Design review of the part built by this model. Coordinates are the model's own, in mm. Face numbers are marked on the shaded views. A direction names the side the tool comes from. Give positions to 0.01 mm unless a question says otherwise; leave off trailing zeros. Write each loop counter-clockwise with the first axis right and the second up, starting at its lowest first coordinate (ties: lowest second). Pieces come first, ordered by that corner, then holes. Notation, with made-up numbers: (34.25, 80.5) -> (41.25, 80.5) arc R21 ccw to (41.25, 107.5) -> close; hole circle Ø8 at (-38.75, 61). An arc over 180 degrees is marked (long way). Return JSON: item names as keys, results as strings. Group by question number.
Autodesk Inventor part; units mm, degrees
ref_plane "Work Plane2" through (0, 3.81, 0) normal (0, 1, 0) x (1, 0, 0)
ref_plane "Work Plane1" through (0, -3.81, 0) normal (0, -1, 0) x (1, 0, 0)
ref_plane "Work Plane4" through (1.27, 3.81, -29.21) normal (0, 0, -1) x (-1, 0, 0)
ref_plane "Work Plane2" through (0, 3.81, 0) normal (0, 1, 0) x (1, 0, 0)
sketch "Sketch2" plane through (0, 3.81, 0) normal (0, 1, 0) x (1, 0, 0)
  line L0 (-29.21, 29.21) -> (1.27, 29.21)
  line L1 (1.27, -1.27) -> (-29.21, -1.27)
  line L2 (-29.21, -1.27) -> (-29.21, 29.21)
  line L3 (1.27, -1.27) -> (1.27, 29.21)
  line L4 (-4.8761, 25.94) -> (-25.94, 25.94)
  line L5 (-25.94, 25.94) -> (-25.94, 0)
  line L6 (-25.94, 0) -> (0, 0)
  line L7 (0, 0) -> (0, 21.0639)
  dimension "d3" = 30.48
extrude "Extrusion2" add sketch "Sketch2" along normal blind 11.43
ref_plane "Work Plane1" through (0, -3.81, 0) normal (0, -1, 0) x (1, 0, 0)
ref_plane "Work Plane4" through (1.27, 3.81, -29.21) normal (0, 0, -1) x (-1, 0, 0)
sketch "Sketch6" plane through (1.27, 3.81, -29.21) normal (0, 0, -1) x (-1, 0, 0)
  line L0 (0, 11.43) -> (30.48, 11.43)
  line L1 (0, 11.43) -> (-7.239, 11.43)
  line L2 (-7.239, 11.43) -> (-7.239, 9.9183)
  line L3 (-7.239, 9.9183) -> (0, 9.9183)
  line L4 (0, 9.9183) -> (0, 11.43)
  line L5 (15.24, 11.43) -> (15.24, -7.62) construction
  line L6 (1.27, -7.62) -> (27.21, -7.62) construction
  line L7 (30.48, 11.43) -> (37.719, 11.43)
  line L8 (37.719, 11.43) -> (37.719, 9.9183)
  line L9 (37.719, 9.9183) -> (30.48, 9.9183)
  line L10 (30.48, 9.9183) -> (30.48, 11.43)
  point P0 (1.27, -3.81)
  dimension "d22" = 7.239
extrude "Extrusion6" add sketch "Sketch6" against normal up to surface (30.48 mm away)
ref_plane "Work Plane3" through (0, 15.24, 0) normal (0, 1, 0) x (1, 0, 0)
sketch "Sketch9" plane through (0, 15.24, 0) normal (0, 1, 0) x (1, 0, 0)
  line L0 (8.509, 29.21) -> (8.509, -1.27) construction
  line L1 (8.509, 13.97) -> (-36.449, 13.97) construction
  line L2 (-36.449, 29.21) -> (-36.449, -1.27) construction
  line L3 (-36.449, -1.27) -> (8.509, -1.27) construction
  line L4 (-13.97, -1.27) -> (-13.97, 29.21) construction
  line L5 (-36.449, 29.21) -> (8.509, 29.21) construction
  circle A0 centre (-21.336, 13.97) radius 3.2512
  circle A1 centre (-6.604, 13.97) radius 3.2512
  line L6 (-6.604, 13.97) -> (-21.336, 13.97) construction
  point P0 (0, 0)
  point P1 (-13.97, 13.97)
  point P2 (-13.97, 13.97)
  point P3 (-13.97, 13.97)
  point P4 (-13.97, 13.97)
  dimension "d25" = 14.732
extrude "Extrusion8" cut sketch "Sketch9" against normal blind 3.2258
ref_plane "Work Plane5" through (0, 15.24, 0) normal (0, 1, 0) x (1, 0, 0)
sketch "Sketch10" plane through (0, 15.24, 0) normal (0, 1, 0) x (1, 0, 0)
  line L0 (-29.21, -1.27) -> (-29.21, 29.21)
  line L1 (1.27, 29.21) -> (1.27, -1.27)
  line L2 (-36.449, 29.21) -> (-36.449, -1.27)
  line L3 (-36.449, 29.21) -> (8.509, 29.21)
  line L4 (-36.449, -1.27) -> (8.509, -1.27)
  line L5 (8.509, 29.21) -> (8.509, -1.27)
  line L6 (-29.21, 29.21) -> (-36.449, 29.21)
  line L7 (-29.21, 29.21) -> (-36.449, 29.21)
  line L8 (-32.8295, 29.21) -> (-32.8295, -1.27)
  line L9 (8.509, 29.21) -> (1.27, 29.21)
  line L10 (4.8895, 29.21) -> (4.8895, -1.27)
  line L11 (8.509, -1.27) -> (4.8895, -1.27)
  line L12 (8.509, 29.21) -> (8.509, -1.27)
  line L13 (8.509, 29.21) -> (8.509, -1.27)
  point P0 (0, 0)
extrude "Extrusion9" cut sketch "Sketch10" against normal blind 25.4 contours L4 L2 L3 L8 | L10 L3 L5 L4
sketch "Sketch18" plane through (0, 3.81, 0) normal (0, -1, 0) x (1, 0, 0)
  line L0 (1.27, 1.27) -> (1.27, -29.21) construction
  line L1 (1.27, -13.97) -> (-29.21, -13.97) construction
  line L2 (-29.21, -29.21) -> (-29.21, 1.27) construction
  line L3 (1.27, -29.21) -> (-29.21, -29.21) construction
  line L4 (-13.97, -29.21) -> (-13.97, 0) construction
  line L5 (0, -13.97) -> (-27.94, -13.97) construction
  line L6 (-13.97, 0) -> (-13.97, -27.94) construction
  line L7 (-13.97, -27.94) -> (-35.862, -27.94) construction
  line L8 (-20.7022, -26.44) -> (-37.4547, -26.44) construction
  line L9 (-27.44, -0.5) -> (-0.5, -0.5)
  line L10 (-0.5, -0.5) -> (-0.5, -27.44)
  line L11 (-0.5, -27.44) -> (-27.44, -27.44)
  line L12 (-27.44, -27.44) -> (-27.44, -0.5)
  line L13 (-27.44, -0.5) -> (-0.5, -27.44) construction
  line L14 (-0.5, -0.5) -> (-27.44, -27.44) construction
  line L15 (-27.44, -8.9624) -> (-18.9776, -0.5)
  point P0 (-13.97, -13.97)
  point P1 (-27.44, -20.8093)
  point P2 (-20.3093, -27.44)
  dimension "d66" = 1.27
  dimension "d72" = 26.94
extrude "Extrusion15" add sketch "Sketch18" along normal blind 7.62
sketch "Sketch19" plane through (0, -3.81, 0) normal (0, -1, 0) x (1, 0, 0)
  line L0 (-2.278, -2.278) -> (-2.278, -25.662) construction
  line L1 (-2.278, -13.97) -> (-25.662, -13.97) construction
  line L2 (-25.662, -25.662) -> (-25.662, -2.278) construction
  line L3 (-25.662, -2.278) -> (-2.278, -2.278) construction
  line L4 (-13.97, -2.278) -> (-13.97, -25.15) construction
  circle A0 centre (-13.97, -13.714) radius 2.0193
  point P0 (0, 0)
  point P1 (-25.412, -19.8229)
  dimension "d79" = 4.0386
extrude "Extrusion16" cut sketch "Sketch19" against normal blind 5.7404
sketch "Sketch21" plane through (0, -3.81, 0) normal (0, -1, 0) x (1, 0, 0)
  line L0 (-0.5, -0.5) -> (-27.44, -0.5)
  line L1 (-27.44, -0.5) -> (-27.44, -27.44)
  line L2 (-25.662, -2.278) -> (-27.44, -0.5)
  line L3 (-27.44, -8.7021) -> (-19.2379, -0.5)
  line L4 (-27.44, -8.7021) -> (-27.44, -0.5)
  point P0 (0, 0)
extrude "Extrusion18" cut sketch "Sketch21" against normal up to surface (7.62 mm away)
chamfer "Chamfer4" distance 1.778 angle 65 5 edges at (-9.869, -3.81, -0.5) (-23.339, -3.81, -4.601) (-27.44, -3.81, -18.071) (-13.97, -3.81, -27.44) (-0.5, -3.81, -13.97) measured on face at (-13.8889, -3.81, -23.5329)
sketch "Sketch22" plane through (0, 15.24, 0) normal (0, 1, 0) x (1, 0, 0)
  line L0 (-29.21, -1.27) -> (-32.8295, -1.27)
  line L1 (-32.8295, -1.27) -> (-29.972, 1.5875)
  line L2 (-32.8295, -1.27) -> (-28.7884, -1.27) construction
  line L3 (-29.6999, -1.27) -> (-32.8295, 1.8596)
  line L4 (-32.8295, -1.27) -> (-32.8295, 29.21)
  line L5 (-32.8295, 1.8596) -> (-32.8295, -1.27)
  point P0 (0, 0)
  dimension "d91" = 45
extrude "Extrusion19" cut sketch "Sketch22" against normal up to surface (1.5117 mm away)
properties part number "IPT_Header" material "Acetal Resin, Black"
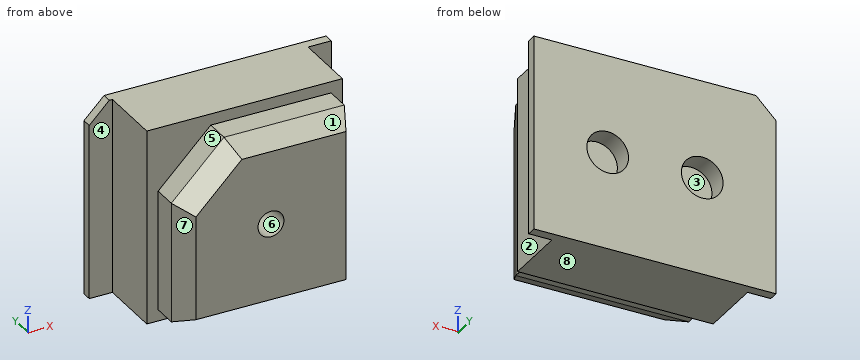
Q1. Tool access review of the marked faces 1, 2, 3, 4 and 5: name each direction out of +Z, -Z, +X, -X, +Y, -Y from which nothing blocks a thin tool from reaching the whole face with its end or side.
Q2. For L1, parallel to X at y = 13, z = -13.97; L2, parallel to Z at x = -13.97, y = 0.35; L3, parallel to X at y = 14.6, z = -13.97, list the stretches that pass through material, from the lowest coordinate up. Write a range as from..to.
Q3. Take a section at B-B, the plane y = 2.5. Give the boundary of the cut face in (x, z).
Q4. Take a section at C-C, the plane x = -11. Give the boundary of the cut face in (y, z), plus the area to 3 significant figures.
Q5. Take a section at D-D, the plane y = 12.75. Give the boundary of the cut face in (x, z).
Q6. Insertion check: pin 1 (8 mm diameter, centred on y = 9.5, z = -21.5, fed in from -X); pin 2 (1.1 mm diameter, centred on y = 2.5, z = -22, fed in from -X); pin 3 (1.1 mm diameter, centred on x = 3, z = -10, fed in from -Y). Each pin has a flat end and moves straight along its axis. Give the tip position at first contact, or say it passes through.
Q7. Mouldability with a two-part tool opening along Z and no side actions: class the marked faces 6, 7 and 8 as +Z half, -Z half, draft (parallel to the pull), parting line (faces both ways), or undercut.
Q8. Take a section at A-A, the plane z = -24. Give the boundary of the cut face in (x, y).
Final values:
{
 "1": {"face 1": "+Z, +X, -X, -Y", "face 2": "+Z, -Z, +X, -Y", "face 3": "+Y", "face 4": "+Z, -Z, -X, -Y", "face 5": "+Z, -X, -Y"},
 "2": {"L1": "x = -29.21..-24.59, -18.08..-9.86, -3.35..1.27", "L2": "z = -27.44..-15.73, -11.69..-0.5", "L3": "x = -32.83..-24.59, -18.08..-9.86, -3.35..4.89"},
 "3": {"outline": "(-27.44, -27.44) -> (-0.5, -27.44) -> (-0.5, -0.5) -> (-19.24, -0.5) -> (-27.44, -8.7) -> close"},
 "4": {"outline": "(-3.81, -25.66) -> (0, -27.44) -> (3.81, -27.44) -> (3.81, -29.21) -> (15.24, -29.21) -> (15.24, 1.27) -> (3.81, 1.27) -> (3.81, -0.5) -> (0, -0.5) -> (-3.81, -2.28) -> close", "area": "547 mm²"},
 "5": {"outline": "(-29.21, -29.21) -> (1.27, -29.21) -> (1.27, 1.27) -> (-29.21, 1.27) -> close; hole circle Ø6.5 at (-21.34, -13.97); hole circle Ø6.5 at (-6.6, -13.97)"},
 "6": {"pin 1": "stops at x = -29.21", "pin 2": "stops at x = -27.44", "pin 3": "stops at y = 13.73"},
 "7": {"face 6": "undercut", "face 7": "draft", "face 8": "-Z half"},
 "8": {"outline": "(-32.83, 13.73) -> (-29.21, 13.73) -> (-29.21, 3.81) -> (-27.44, 3.81) -> (-27.44, 0) -> (-25.66, -3.81) -> (-2.28, -3.81) -> (-0.5, 0) -> (-0.5, 3.81) -> (1.27, 3.81) -> (1.27, 13.73) -> (4.89, 13.73) -> (4.89, 15.24) -> (-32.83, 15.24) -> close"}
}
